For this review, take the finished solid that the model builds, in its own axes (mm). A direction names the side the tool comes from. Round coordinates to 2 decimals unless told otherwise and drop trailing zeros. Loops run counter-clockwise (first coordinate to the right, second up) from the corner with the lowest first, then second, coordinate; pieces in that order, holes last. Notation, with made-up numbers: (-34.75, -26.5) -> (-30.75, -26.5) arc R21 cw to (-30.75, -3.5) -> close; hole circle Ø9 at (14.25, 55.25). An arc over 180 degrees is marked (long way). One line per question, with ' | ' between items. Start each with the question number.
1. Consider section B-B (x = 19.05). Write out the cut boundary in (y, z), and give its area (3 significant figures).
2. For pin 1 Ø8 at (x, z) = (39, -18.5) entering from +Y; pin 2 Ø20.5 at (x, z) = (-38.1, 19.05) entering from -Y; pin 3 Ø4 at (x, z) = (38.1, -57.15) entering from +Y; pin 4 Ø6.5 at (x, z) = (-14.5, 5) entering from -Y, all flat-tipped, find the tip position at first contact; note any pin that passes through.
3. Consider section D-D (z = 19.05). Write out the cut boundary in (x, y) (1 decimal).
4. Wall thickness on line 1 along Z through (x, y) = (38.1, -2.1); line 2 along Z through (x, y) = (38.1, -6.5) (3 decimals); line 3 along X through (y, z) = (-1.5, 18): over which ranges is each line inside the solid? List them lowest first.
5. Draft analysis for pull direction Z (two halves, no side actions). For faces 1 (the face through (-1, -12.7, 1)), 2 (the face through (-1, -6, 76.2)), 3 (the face through (-14, -7.937, 51)), state which applies: pulls with the +Z half, pulls with the -Z half, needs draft (parallel to the pull), parting line crosses it, or undercut.
6. For faces 4 (the face through (-30.17, -2.46, -18.7)), 5 (the face through (-14, -7.937, -51)), 6 (the face through (14.292, -4.024, 0.209)), list the 3-axis set-ups (+Z, -Z, +X, -X, +Y, -Y) from which the entire face can be reached by the end or side of a thin tool; tool diameter is ignored.
7. Consider section A-A (z = 0). Write out the cut boundary in (x, y), and give its area (3 significant figures).
8. Consider section C-C (y = -9.5). Count the separate pieces of the cut face and the enclosed holes in it, and give its area (3 significant figures).
```python
from build123d import *

# Parameters (mm, degrees)
F0_W     = 101.6
F0_H     = 152.4
F1_DEPTH = 12.7
F2_R     = 3.175
F3_DEPTH = 12.701
F4_R     = 7.9375
F5_DEPTH = 5
F6_R     = 4.7625
F7_DEPTH = 12.701
F8_R     = 11.1125
F9_DEPTH = 4.7625


with BuildPart() as f1:
    # F0 (on Front) → F1 (new body)
    with BuildSketch(Plane.XZ):
        Rectangle(F0_W, F0_H)
    extrude(amount=F1_DEPTH)

    # F2 (on face) → F3 (cut, through all)
    with BuildSketch(Plane.XZ.offset(12.7)):
        with Locations((-38.1, 57.15)):
            Circle(F2_R)
        with Locations((-38.1, 19.05)):
            Circle(F2_R)
        with Locations((-38.1, -19.05)):
            Circle(F2_R)
        with Locations((-38.1, -57.15)):
            Circle(F2_R)
        with Locations((38.1, 57.15)):
            Circle(F2_R)
        with Locations((38.1, 19.05)):
            Circle(F2_R)
        with Locations((38.1, -19.05)):
            Circle(F2_R)
        with Locations((38.1, -57.15)):
            Circle(F2_R)
    extrude(amount=-F3_DEPTH, mode=Mode.SUBTRACT)

    # F4 (on face) → F5 (cut)
    with BuildSketch(Plane(origin=(0, 0, 0), x_dir=(-1, 0, 0), z_dir=(0, 1, 0))):
        with Locations((-38.1, 57.15)):
            Circle(F4_R)
        with Locations((-38.1, 19.05)):
            Circle(F4_R)
        with Locations((-38.1, -19.05)):
            Circle(F4_R)
        with Locations((-38.1, -57.15)):
            Circle(F4_R)
        with Locations((38.1, 57.15)):
            Circle(F4_R)
        with Locations((38.1, 19.05)):
            Circle(F4_R)
        with Locations((38.1, -19.05)):
            Circle(F4_R)
        with Locations((38.1, -57.15)):
            Circle(F4_R)
    extrude(amount=-F5_DEPTH, mode=Mode.SUBTRACT)

    # F6 (on face) → F7 (cut, through all)
    with BuildSketch(Plane.XZ.offset(12.7)):
        with Locations((-19.05, 50.8)):
            Circle(F6_R)
        with Locations((-19.05, 0)):
            Circle(F6_R)
        with Locations((-19.05, -50.8)):
            Circle(F6_R)
        with Locations((19.05, 50.8)):
            Circle(F6_R)
        with Locations((19.05, 0)):
            Circle(F6_R)
        with Locations((19.05, -50.8)):
            Circle(F6_R)
    extrude(amount=-F7_DEPTH, mode=Mode.SUBTRACT)

    # F8 (on face) → F9 (cut)
    with BuildSketch(Plane.XZ.offset(12.7)):
        with Locations((-19.05, 50.8)):
            Circle(F8_R)
        with Locations((-19.05, 0)):
            Circle(F8_R)
        with Locations((-19.05, -50.8)):
            Circle(F8_R)
        with Locations((19.05, 50.8)):
            Circle(F8_R)
        with Locations((19.05, 0)):
            Circle(F8_R)
        with Locations((19.05, -50.8)):
            Circle(F8_R)
    extrude(amount=-F9_DEPTH, mode=Mode.SUBTRACT)


solid = f1.part
```
Answer block:
1) outline: (-12.7, -76.2) -> (0, -76.2) -> (0, -55.56) -> (-7.94, -55.56) -> (-7.94, -61.91) -> (-12.7, -61.91) -> close; (-12.7, -39.69) -> (-7.94, -39.69) -> (-7.94, -46.04) -> (0, -46.04) -> (0, -4.76) -> (-7.94, -4.76) -> (-7.94, -11.11) -> (-12.7, -11.11) -> close; (-12.7, 11.11) -> (-7.94, 11.11) -> (-7.94, 4.76) -> (0, 4.76) -> (0, 46.04) -> (-7.94, 46.04) -> (-7.94, 39.69) -> (-12.7, 39.69) -> close; (-12.7, 61.91) -> (-7.94, 61.91) -> (-7.94, 55.56) -> (0, 55.56) -> (0, 76.2) -> (-12.7, 76.2) -> close | area: 1,390 mm2
2) pin 1: stops at y = -5 | pin 2: stops at y = -12.7 | pin 3: passes through | pin 4: stops at y = -7.94
3) outline: (-50.8, -12.7) -> (-41.3, -12.7) -> (-41.3, -5) -> (-46, -5) -> (-46, 0) -> (-50.8, 0) -> close; (-34.9, -12.7) -> (34.9, -12.7) -> (34.9, -5) -> (30.2, -5) -> (30.2, 0) -> (-30.2, 0) -> (-30.2, -5) -> (-34.9, -5) -> close; (41.3, -12.7) -> (50.8, -12.7) -> (50.8, 0) -> (46, 0) -> (46, -5) -> (41.3, -5) -> close
4) line 1: z = -76.2 to -65.09, -49.21 to -26.99, -11.11 to 11.11, 26.99 to 49.21, 65.09 to 76.2 | line 2: z = -76.2 to -60.325, -53.975 to -22.225, -15.875 to 15.875, 22.225 to 53.975, 60.325 to 76.2 | line 3: x = -50.8 to -45.97, -30.23 to 30.23, 45.97 to 50.8
5) face 1: needs draft | face 2: pulls with the +Z half | face 3: undercut
6) face 4: +Y | face 5: -Y | face 6: +Y, -Y
7) outline: (-50.8, -12.7) -> (-30.16, -12.7) -> (-30.16, -7.94) -> (-23.81, -7.94) -> (-23.81, 0) -> (-50.8, 0) -> close; (-14.29, -7.94) -> (-7.94, -7.94) -> (-7.94, -12.7) -> (7.94, -12.7) -> (7.94, -7.94) -> (14.29, -7.94) -> (14.29, 0) -> (-14.29, 0) -> close; (23.81, -7.94) -> (30.16, -7.94) -> (30.16, -12.7) -> (50.8, -12.7) -> (50.8, 0) -> (23.81, 0) -> close | area: 927 mm2
8) separate pieces: 1 | enclosed holes: 14 | area: 12,900 mm2
